Read the model definition and answer for the solid it produces. Units are mm, in the model's axes. A direction names the side the tool comes from. Give positions to 0.01 mm unless a question says otherwise; leave off trailing zeros. Order: outer loops, then holes, each group sorted by start corner. A loop starts at its lowest first (then second) coordinate and runs counter-clockwise, first axis right, second up. Notation, with made-up numbers: (-39.5, -37.5) - (11.5, -37.5) arc R18 ccw to (11.5, -8.5) - close; hole circle Ø4 at (30, -38.75). An arc over 180 degrees is marked (long way). Write each question's results on one line, items separated by ' | '.
from build123d import *
from OCP.BRepFilletAPI import BRepFilletAPI_MakeChamfer

# Parameters (mm, degrees)
BOSS_EXTRUDE1_DEPTH      = 3.8
BOSS_EXTRUDE1_DEPTH_BACK = 3
SKETCH1_W                = 38
SKETCH1_H                = 40
SKETCH1_R                = 4.15
BOSS_EXTRUDE2_DEPTH      = 3
FILLET1_R                = 3
SKETCH3_W                = 9.5
SKETCH3_H                = 4
BOSS_EXTRUDE3_DEPTH      = 4
BOSS_EXTRUDE4_DEPTH      = 2.9
CHAMFER1_SIZE            = 3
CHAMFER1_SIZE2           = 2.307927774


with BuildPart() as part:
    # Sketch1 → Boss-Extrude1 (new, two sides: drawn at the far end of the back side and taken through both)
    with BuildSketch(Plane.XY.offset(-BOSS_EXTRUDE1_DEPTH_BACK)):
        Rectangle(SKETCH1_W, SKETCH1_H)
        with Locations(Location((0, 0, 0), (0, 0, 180))):
            Circle(SKETCH1_R, mode=Mode.SUBTRACT)
    extrude(amount=BOSS_EXTRUDE1_DEPTH + BOSS_EXTRUDE1_DEPTH_BACK)

    # Sketch2 → Boss-Extrude2 (add)
    with BuildSketch(Plane.XY):
        Polygon((5, 20), (5, 22), (-5, 47), (-5, 20), align=None)
    extrude(amount=-BOSS_EXTRUDE2_DEPTH)

    # Fillet1
    # the kernel refuses this fillet: 3 mm, written as the material it adds along each edge
    with BuildSketch(Plane(origin=(-5, 20, 0), x_dir=(-1, 0, 0), z_dir=(0, 0, -1))) as fillet1_piece_1:
        with BuildLine():
            CenterArc((FILLET1_R, FILLET1_R), FILLET1_R, 180, 90)
            Line((0, FILLET1_R), (0, 0))
            Line((0, 0), (FILLET1_R, 0))
        make_face()
    extrude(amount=3)
    with BuildSketch(Plane(origin=(5, 20, 0), x_dir=(1, 0, 0), z_dir=(0, 0, -1))) as fillet1_piece_2:
        with BuildLine():
            CenterArc((2.828427125, -3), FILLET1_R, 90, 70.528779366)
            Line((0, -2), (0, 0))
            Line((0, 0), (2.828427125, 0))
        make_face()
    extrude(amount=3)
    # the kernel refuses this fillet: 3 mm, written as the material it takes off along each edge
    with BuildSketch(Plane(origin=(19, -20, -10.5), x_dir=(-1, 0, 0), z_dir=(0, 0, 1)), Plane(origin=(-19, -20, 11.3), x_dir=(1, 0, 0), z_dir=(0, 0, -1))) as fillet1_2_piece_1:
        with BuildLine():
            CenterArc((FILLET1_R, -FILLET1_R), FILLET1_R, 90, 90)
            Line((0, -FILLET1_R), (0, 0))
            Line((0, 0), (FILLET1_R, 0))
        make_face()
    extrude(amount=21.8, mode=Mode.SUBTRACT)

    # Sketch3 → Boss-Extrude3 (add)
    with BuildSketch(Plane.XY.offset(3.8)):
        with Locations((0, -15)):
            Rectangle(SKETCH3_W, SKETCH3_H)
        with Locations((0, 15)):
            Rectangle(SKETCH3_W, SKETCH3_H)
    extrude(amount=BOSS_EXTRUDE3_DEPTH)

    # Sketch4 → Boss-Extrude4 (add)
    with BuildSketch(Plane.XY):
        Polygon((-5, 29.2), (2.12, 29.2), (-5, 47), align=None)
    extrude(amount=BOSS_EXTRUDE4_DEPTH)

    # Chamfer1: one chamfer whose edges measure the first distance from different faces: ONE call of the kernel's chamfer builder (chamfer() names one face for all edges)
    chamfer1_edges_1 = [part.edges().sort_by_distance(p)[0] for p in [
        (-5, 29.2, 1.45),
        (4.75, 15, 7.8),
        (-4.75, 15, 7.8),
        (4.75, -15, 7.8),
        (-4.75, -15, 7.8),
    ]]
    chamfer1_edges_2 = [part.edges().sort_by_distance(p)[0] for p in [
        (2.12, 29.2, 1.45),
    ]]
    chamfer1_side_2 = [part.faces().sort_by_distance(p)[0] for p in [
        (-1.44, 29.2, 1.45),
    ]]
    chamfer1 = BRepFilletAPI_MakeChamfer(part.part.solid().wrapped)
    for e in chamfer1_edges_1:
        chamfer1.Add(CHAMFER1_SIZE, e.wrapped)
    for e in chamfer1_edges_2:
        chamfer1.Add(CHAMFER1_SIZE, CHAMFER1_SIZE2, e.wrapped, chamfer1_side_2[0].wrapped)  # the first distance lies on this face
    add(Compound.cast(chamfer1.Shape()), mode=Mode.REPLACE)


solid = part.part
(1) For faces 4 (the face through (0, -17, 5)), 5 (the face through (-3, 36, 2.9)), 6 (the face through (0, -13, 5)), determine the directions among +Z, -Z, +X, -X, +Y, -Y from which every point of the face is accessible in a straight line to the end or side of a thin tool.
Conclusion:
face 4: +Z, +X, -X, -Y | face 5: +Z, +X, -X, +Y | face 6: +Z, +X, -X
(2) Section D-D (y = 28) is taken. Give the vertices of the cut face in (x, z), plus the area to 3 significant figures.
Conclusion:
outline: (-5, -3) - (2.6, -3) - (2.6, 0) - (-5, 0) - close | area: 22.8 mm^2
(3) Each of these flat-tipped pins is pushed along its axis until it touches: pin 1 (5 mm diameter, centred on y = 26.5, z = 6, fed in from -X); pin 2 (1.9 mm diameter, centred on x = -2, y = 36.5, fed in from +Z); pin 3 (3.5 mm diameter, centred on x = -1, y = 26.5, fed in from +Z); pin 4 (4.5 mm diameter, centred on y = 37.5, z = 1, fed in from -X). Where does it stop, or does it pass through?
Conclusion:
pin 1: through | pin 2: z = 2.9 | pin 3: z = 0 | pin 4: x = -5
(4) Section C-C (y = 0) is taken. Give the vertices of the cut face in (x, z), plus the area to 3 significant figures.
Conclusion:
outline: (-19, -3) - (-4.15, -3) - (-4.15, 3.8) - (-19, 3.8) - close; (4.15, -3) - (19, -3) - (19, 3.8) - (4.15, 3.8) - close | area: 202 mm^2
(5) Section A-A (z = 6.5) is taken. Give the vertices of the cut face in (x, y), plus the area to 3 significant figures.
Conclusion:
outline: (-3.05, -17) - (3.05, -17) - (3.05, -13) - (-3.05, -13) - close; (-3.05, 13) - (3.05, 13) - (3.05, 17) - (-3.05, 17) - close | area: 48.8 mm^2
(6) Section B-B (x = 0) is taken. Give the vertices of the cut face in (y, z).
Conclusion:
outline: (-20, -3) - (-4.15, -3) - (-4.15, 3.8) - (-13, 3.8) - (-13, 7.8) - (-17, 7.8) - (-17, 3.8) - (-20, 3.8) - close; (4.15, -3) - (34.5, -3) - (34.5, 2.9) - (30.08, 2.9) - (30.08, 0) - (20, 0) - (20, 3.8) - (17, 3.8) - (17, 7.8) - (13, 7.8) - (13, 3.8) - (4.15, 3.8) - close
(7) The mould has two halves that part along Y. Classify faces 1 (the face through (0, 17, 5)), 2 (the face through (-18.1, -19.14, 0.45)), 3 (the face through (0, 13, 5)): pulls with the +Y half, pulls with the -Y half, needs draft (parallel to the pull), parting line crosses it, or undercut.
Conclusion:
face 1: pulls with the +Y half | face 2: pulls with the -Y half | face 3: undercut
(8) Consider probe 1 along Y at (x, z) = (-4, 4); probe 2 along Z at (x, y) = (6, -9.5); probe 3 along X at (y, z) = (-2, -1.25). Determine where each line is inside the solid, lowest interval first. Write a range as [from, to].
Conclusion:
probe 1: [-17, -13], [13, 17] | probe 2: [-3, 3.8] | probe 3: [-19, -3.64], [3.64, 19]
